Model file for the job. Use its own axes, mm. Face numbers are marked on the shaded views. A direction names the side the tool comes from. Give positions to 0.01 mm unless a question says otherwise; leave off trailing zeros. Loops run counter-clockwise (first coordinate to the right, second up) from the corner with the lowest first, then second, coordinate; pieces in that order, holes last. Notation, with made-up numbers: (9.25, 35) - (21.25, 35) arc R18 cw to (21.25, 55) - close; hole circle Ø2 at (-34, -15). An arc over 180 degrees is marked (long way). Use a Markdown table: item, result.
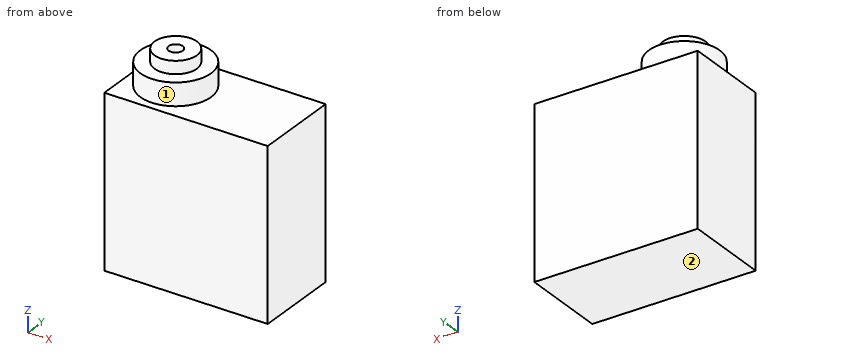
from build123d import *

# Parameters (mm, degrees)
SKETCH_1_W          = 23.1
SKETCH_1_H          = 12.2
EXTRUDE_1_DEPTH     = 27.1
SKETCH_2_R          = 5
EXTRUDE_2_DEPTH     = 3.2
SKETCH_3_W          = 23.1
SKETCH_3_H          = 12.2
CUT_EXTRUDE_1_DEPTH = 3.2
SKETCH_4_R          = 3
CUT_EXTRUDE_2_DEPTH = 3.2
EXTRUDE_START       = 4.995444433
SKETCH_5_R          = 3
EXTRUDE_3_DEPTH     = 4.995444433
SKETCH_7_R          = 1
CUT_EXTRUDE_3_DEPTH = 5


with BuildPart() as part:
    # 草图1 → 凸台-拉伸1 (new body)
    with BuildSketch(Plane.XY):
        with Locations((-0.26021144, -3.034725608)):
            Rectangle(SKETCH_1_W, SKETCH_1_H)
    extrude(amount=-EXTRUDE_1_DEPTH)

    # 草图2 → 凸台-拉伸2 (add)
    with BuildSketch(Plane.XY):
        with Locations((-5.81021144, -3.034725608)):
            Circle(SKETCH_2_R)
    extrude(amount=EXTRUDE_2_DEPTH)

    # 草图3 → 切除-拉伸1 (cut)
    with BuildSketch(Plane(origin=(0, 0, -27.1), x_dir=(-1, 0, 0), z_dir=(0, 0, -1))):
        with Locations((0.26021144, -3.034725608)):
            Rectangle(SKETCH_3_W, SKETCH_3_H)
    extrude(amount=-CUT_EXTRUDE_1_DEPTH, mode=Mode.SUBTRACT)

    # 草图4 → 切除-拉伸2 (cut)
    with BuildSketch(Plane.XY.offset(3.2)):
        with Locations((-5.81021144, -3.034725608)):
            Circle(SKETCH_4_R)
    extrude(amount=-CUT_EXTRUDE_2_DEPTH, mode=Mode.SUBTRACT)

    # 草图5 → 凸台-拉伸3 (add)
    with BuildSketch(Plane.XY.offset(EXTRUDE_START)):
        with Locations((-5.81021144, -3.034725608)):
            Circle(SKETCH_5_R)
    extrude(amount=-EXTRUDE_3_DEPTH)

    # 草图7 → 切除-拉伸3 (cut)
    with BuildSketch(Plane.XY.offset(4.995444433)):
        with Locations((-5.81021144, -3.034725608)):
            Circle(SKETCH_7_R)
    extrude(amount=-CUT_EXTRUDE_3_DEPTH, mode=Mode.SUBTRACT)


solid = part.part
(1) Slice it at A-A, the plane x = 4.25. Write the cut outline in (y, z).
Computed:
| item | result |
|---|---|
| outline | (-9.13, -23.9) - (3.07, -23.9) - (3.07, 0) - (-9.13, 0) - close |
(2) Slice it at C-C, the plane x = -2. Write the cut outline in (y, z).
Computed:
| item | result |
|---|---|
| outline | (-9.13, -23.9) - (3.07, -23.9) - (3.07, 0) - (0.2, 0) - (0.2, 3.2) - (-6.27, 3.2) - (-6.27, 0) - (-9.13, 0) - close |
(3) 3-axis set-ups, long thin cutter, end or side, ignore diameter. For the marked faces 1 and 2: which of +Z, -Z, +X, -X, +Y, -Y reach the whole face in a straight line?
Computed:
| item | result |
|---|---|
| face 1 | +Z |
| face 2 | -Z, +X, -X, +Y, -Y |
(4) Drill centre lines: probe 1 along Z at (x, y) = (7, -3); probe 2 along Z at (x, y) = (-6, -7.75); probe 3 along X at (y, z) = (-2.5, 2.5). Where is each one in solid material? Low to high. Write a range as [from, to].
Computed:
| item | result |
|---|---|
| probe 1 | [-23.9, 0] |
| probe 2 | [-23.9, 3.2] |
| probe 3 | [-10.78, -6.66], [-4.97, -0.84] |
(5) Slice it at B-B, the plane y = -1.5. Write the cut outline in (x, z).
Computed:
| item | result |
|---|---|
| outline | (-11.81, -23.9) - (11.29, -23.9) - (11.29, 0) - (-1.05, 0) - (-1.05, 3.2) - (-3.23, 3.2) - (-3.23, 5) - (-8.39, 5) - (-8.39, 3.2) - (-10.57, 3.2) - (-10.57, 0) - (-11.81, 0) - close |
(6) Slice it at D-D, the plane x = -5.5. Write the cut outline in (y, z), plus the area to 3 significant figures.
Computed:
| item | result |
|---|---|
| outline | (-9.13, -23.9) - (3.07, -23.9) - (3.07, 0) - (1.96, 0) - (1.96, 3.2) - (-0.05, 3.2) - (-0.05, 5) - (-2.08, 5) - (-2.08, 0) - (-3.99, 0) - (-3.99, 5) - (-6.02, 5) - (-6.02, 3.2) - (-8.03, 3.2) - (-8.03, 0) - (-9.13, 0) - close |
| area | 325 mm² |
